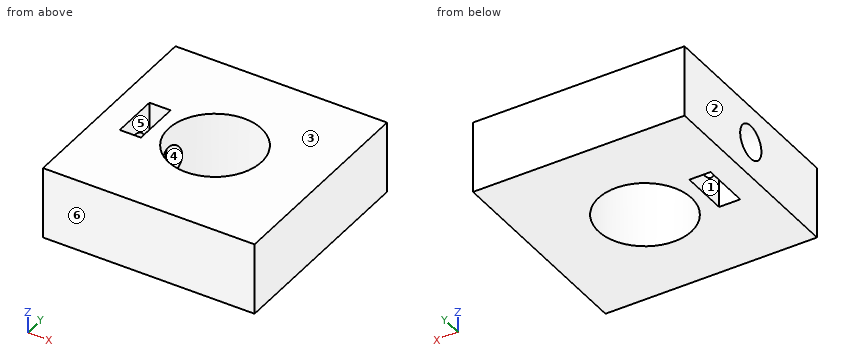
from build123d import *

# Parameters (mm, degrees)
SKETCH002_W         = 2.5
SKETCH002_H         = 5.6
EXTRUDE002_DEPTH    = 10
SKETCH001_R         = 2
EXTRUDE001_DEPTH    = 10
SKETCH_W            = 25
SKETCH_H            = 25
SKETCH_R            = 5.5
EXTRUDE_DEPTH       = 8.5
CUT_PLACEMENT_ANGLE = 180


with BuildPart() as extrude002:
    # Sketch002 → Extrude002 (new body)
    with BuildSketch(Plane.XY):
        with Locations((-8.25, 0)):
            Rectangle(SKETCH002_W, SKETCH002_H)
    extrude(amount=EXTRUDE002_DEPTH)


with BuildPart() as extrude002_1:
    # Extrude002 placement: moved
    add(extrude002.part.moved(Location((0, 0, -1))))


with BuildPart() as extrude001:
    # Sketch001 → Extrude001 (new body)
    with BuildSketch(Plane.YZ.offset(12.5)):
        with Locations((0, 4.2)):
            Circle(SKETCH001_R)
    extrude(amount=EXTRUDE001_DEPTH)


with BuildPart() as extrude001_1:
    # Extrude001 placement: moved
    add(extrude001.part.moved(Location((-8, 0, 0))))


with BuildPart() as cut001:
    # Sketch → Extrude (new body)
    with BuildSketch(Plane.XY):
        Rectangle(SKETCH_W, SKETCH_H)
        Circle(SKETCH_R, mode=Mode.SUBTRACT)
    extrude(amount=EXTRUDE_DEPTH)

    # Cut: cut Extrude001
    add(extrude001_1.part, mode=Mode.SUBTRACT)


with BuildPart() as cut001_1:
    # Cut placement: moved
    add(cut001.part.rotate(Axis((0, 0, 0), (0, 0, 1)), CUT_PLACEMENT_ANGLE))

    # Cut001: cut Extrude002
    add(extrude002_1.part, mode=Mode.SUBTRACT)


solid = cut001_1.part
Read the model definition and answer for the solid it produces. Units are mm, in the model's axes. Face numbers are marked on the shaded views. A direction names the side the tool comes from. Coordinates: 2 decimals unless noted, no trailing zeros. Loops run counter-clockwise (first coordinate to the right, second up) from the corner with the lowest first, then second, coordinate; pieces in that order, holes last.
Q1. Which of the six approach directions +Z, -Z, +X, -X, +Y, -Y give full straight-line access (tool end or side, diameter ignored) to the marked faces 4, 5 and 6?
Q2. The part is cut by section A-A on x = 0. Write down the section's boundary in (y, z), and give its area (3 significant figures).
Q3. The part is cut by section B-B on z = 7.75. Write down the section's boundary in (x, y).
Q4. Each of these flat-tipped pins is pushed along its axis until it touches: pin 1 Ø12 at (x, y) = (-7.5, 1) entering from -Z; pin 2 Ø6.5 at (x, y) = (0, 0) entering from -Z. Where does it stop, or does it pass through?
Q5. The mould has two halves that part along X. Classify the marked faces 1, 2 and 3: +X half, -X half, draft (parallel to the pull), parting line (faces both ways), or undercut.
Q6. The part is cut by section D-D on x = -10.5. Write down the section's boundary in (y, z).
Q7. The part is cut by section C-C on y = 0. Write down the section's boundary in (x, z).
Q8. Consider probe 1 along Z at (x, y) = (-10.2, 0); probe 2 along Y at (x, z) = (-6.1, 4.2); probe 3 along X at (y, z) = (-2.5, 8). Determine where each line is inside the solid, lowest interval first.
Results below:
1. face 4: -X
1. face 5: +Z, -Z
1. face 6: +Z, -Z, +X, -X, -Y
2. outline: (-12.5, 0) - (-5.5, 0) - (-5.5, 8.5) - (-12.5, 8.5) - close; (5.5, 0) - (12.5, 0) - (12.5, 8.5) - (5.5, 8.5) - close
2. area: 119 mm2
3. outline: (-12.5, -12.5) - (12.5, -12.5) - (12.5, 12.5) - (-12.5, 12.5) - close; hole (-9.5, -2.8) - (-7, -2.8) - (-7, 2.8) - (-9.5, 2.8) - close; hole circle Ø11 at (0, 0)
4. pin 1: stops at z = 0
4. pin 2: passes through
5. face 1: undercut
5. face 2: -X half
5. face 3: draft
6. outline: (-12.5, 0) - (12.5, 0) - (12.5, 8.5) - (-12.5, 8.5) - close; hole circle Ø4 at (0, 4.2)
7. outline: (-12.5, 0) - (-9.5, 0) - (-9.5, 2.2) - (-12.5, 2.2) - close; (-12.5, 6.2) - (-9.5, 6.2) - (-9.5, 8.5) - (-12.5, 8.5) - close; (-7, 0) - (-5.5, 0) - (-5.5, 2.2) - (-7, 2.2) - close; (-7, 6.2) - (-5.5, 6.2) - (-5.5, 8.5) - (-7, 8.5) - close; (5.5, 0) - (12.5, 0) - (12.5, 8.5) - (5.5, 8.5) - close
8. probe 1: z = 0 to 2.2, 6.2 to 8.5
8. probe 2: y = -12.5 to -2, 2 to 12.5
8. probe 3: x = -12.5 to -9.5, -7 to -4.9, 4.9 to 12.5
